Answer from the drawing. Dimensions are ordinates in mm from the lowest x, y and z of the part. A direction names the side the tool comes from. Round coordinates to 2 decimals unless told otherwise and drop trailing zeros. Order: outer loops, then holes, each group sorted by start corner. A loop starts at its lowest first (then second) coordinate and runs counter-clockwise, first axis right, second up. Notation, with made-up numbers: (21.25, 11.5) - (76.25, 11.5) arc R23 ccw to (76.25, 47.5) - close; hole circle Ø10 at (-21.75, 74). An arc over 180 degrees is marked (long way). One line per question, with ' | ' between items. Start each with the question number.
1) The mould has two halves that part along Z. Classify the marked faces 1, 2, 3 and 4: pulls with the +Z half, pulls with the -Z half, needs draft (parallel to the pull), parting line crosses it, or undercut.
2) The part is cut by section C-C, the plane y = 0.4. Give the vertices of the cut face in (x, z).
3) For the marked faces 5 and 6, determine the directions among +Z, -Z, +X, -X, +Y, -Y from which every point of the face is accessible in a straight line to the end or side of a thin tool.
4) The part is cut by section A-A, the plane y = 2. Give the vertices of the cut face in (x, z).
5) The part is cut by section B-B, the plane z = 2.9. Give the vertices of the cut face in (x, y).
6) The part is cut by section D-D, the plane x = 1.4. Give the vertices of the cut face in (y, z).
7) Straight lines are drawn through the part: line 1 (Y direction, x = 0.4, z = 2.95); line 2 (X direction, y = 0.45, z = 1.05); line 3 (Z direction, x = 0.7, y = 2). For each, find the intervals that lie inside material, in ascending order. Write a range as from..to.
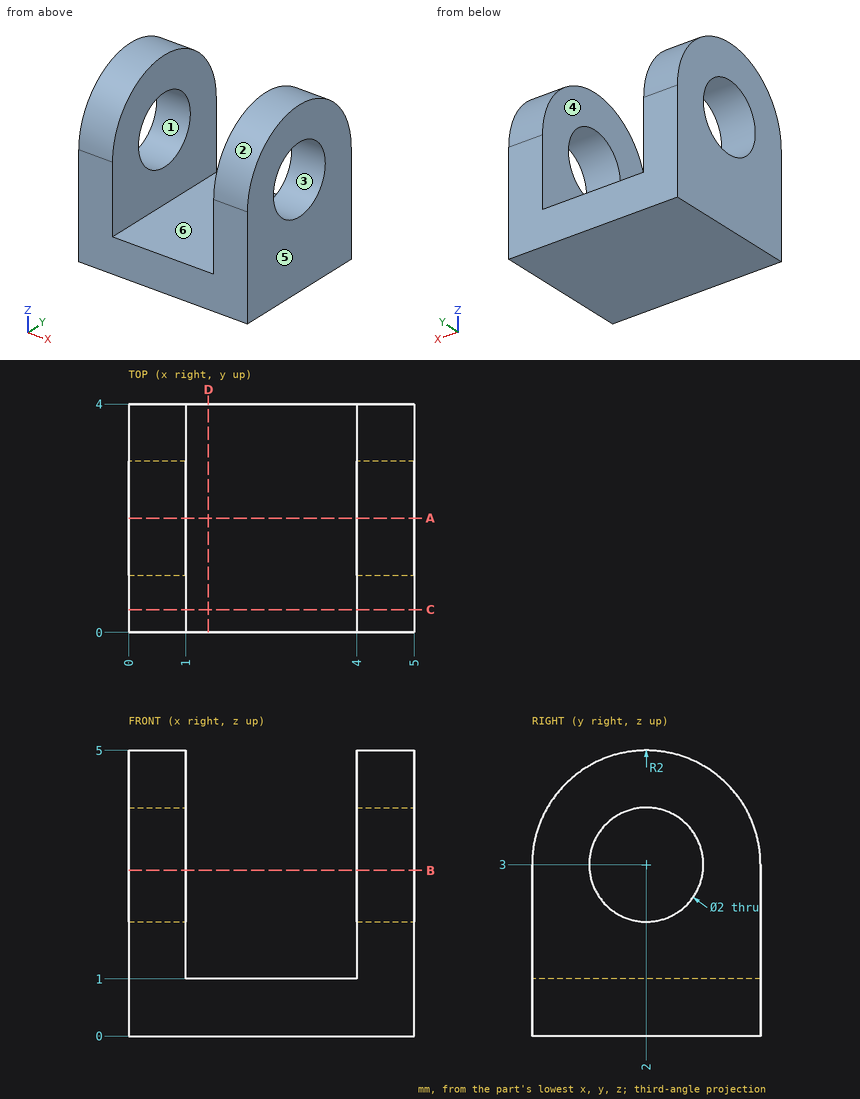
Values:
1) face 1: undercut | face 2: pulls with the +Z half | face 3: undercut | face 4: needs draft
2) outline: (0, 0) - (5, 0) - (5, 4.2) - (4, 4.2) - (4, 1) - (1, 1) - (1, 4.2) - (0, 4.2) - close
3) face 5: +Z, -Z, +X, +Y, -Y | face 6: +Z, +Y, -Y
4) outline: (0, 0) - (5, 0) - (5, 2) - (4, 2) - (4, 1) - (1, 1) - (1, 2) - (0, 2) - close; (0, 4) - (1, 4) - (1, 5) - (0, 5) - close; (4, 4) - (5, 4) - (5, 5) - (4, 5) - close
5) outline: (0, 0) - (1, 0) - (1, 1.01) - (0, 1.01) - close; (0, 2.99) - (1, 2.99) - (1, 4) - (0, 4) - close; (4, 0) - (5, 0) - (5, 1.01) - (4, 1.01) - close; (4, 2.99) - (5, 2.99) - (5, 4) - (4, 4) - close
6) outline: (0, 0) - (4, 0) - (4, 1) - (0, 1) - close
7) line 1: y = 0..1, 3..4 | line 2: x = 0..1, 4..5 | line 3: z = 0..2, 4..5
